Can you work these out from the model? Positions are in its coordinate system, mm. A direction names the side the tool comes from. Round coordinates to 2 decimals unless told otherwise and drop trailing zeros. Loops run counter-clockwise (first coordinate to the right, second up) from the corner with the lowest first, then second, coordinate; pieces in that order, holes last. Notation, with made-up numbers: (11.25, -1.5) -> (40.25, -1.5) arc R22 cw to (40.25, 35.5) -> close; hole circle Ø3 at (-37, 57). An arc over 180 degrees is marked (long way). Write each question's results on one line, items separated by ' | '.
from build123d import *

# Parameters (mm, degrees)
F0_R     = 17.5
F1_DEPTH = 4.9
F2_R     = 30
F3_DEPTH = 6.6
F4_SIZE  = 2
F5_R     = 7.5
F5_R_2   = 4.075
F6_DEPTH = 7.7
F7_DEPTH = 11.501


with BuildPart() as f1:
    # F0 (on Top) → F1 (new body)
    with BuildSketch(Plane.XY):
        Circle(F0_R)
    extrude(amount=F1_DEPTH)

    # F2 (on face) → F3 (join)
    with BuildSketch(Plane.XY.offset(4.9)):
        Circle(F2_R)
    extrude(amount=F3_DEPTH)

    # F4
    f4_edges = [f1.edges().sort_by_distance(p)[0] for p in [
        (-30, 0, 11.5),
    ]]
    chamfer(f4_edges, length=F4_SIZE)

    # F5 (on face) → F6 (cut)
    with BuildSketch(Plane.XY.offset(11.5)):
        with Locations((-8.8, 0)):
            Circle(F5_R)
        with Locations((-8.8, 0)):
            Circle(F5_R_2, mode=Mode.SUBTRACT)
        with Locations((8.8, 0)):
            Circle(F5_R)
        with Locations((8.8, 0)):
            Circle(F5_R_2, mode=Mode.SUBTRACT)
    extrude(amount=-F6_DEPTH, mode=Mode.SUBTRACT)

    # F7 (cut, through all): faces of the model
    f7_faces = [f1.faces().sort_by_distance(p)[0] for p in [
        (-8.8, 0, 11.5),
        (8.8, 0, 11.5),
    ]]
    extrude(f7_faces, amount=-F7_DEPTH, mode=Mode.SUBTRACT)


solid = f1.part
1. On a 3-axis mill with a long thin cutter (end or side, diameter ignored), from which of +Z, -Z, +X, -X, +Y, -Y can I reach the whole of each face in a straight line? I mean faces 1 (the face through (-29.97, 1.32, 7.17)), 2 (the face through (15.73, -2.87, 7.7)), 3 (the face through (13, -13, 4.9)). Say none if no direction works.
Final values:
face 1: +Z, -Z | face 2: +Z | face 3: -Z
2. If we section it at A-A (x = 0): List the corners of the cut face in (y, z) for me.
Final values:
outline: (-30, 4.9) -> (-17.5, 4.9) -> (-17.5, 0) -> (17.5, 0) -> (17.5, 4.9) -> (30, 4.9) -> (30, 9.5) -> (28, 11.5) -> (-28, 11.5) -> (-30, 9.5) -> close
3. If we section it at C-C (z = 8.25): List the corners of the cut face in (x, y) for me, then the cut area to 3 significant figures.
Final values:
outline: circle Ø60 at (0, 0); hole circle Ø15 at (-8.8, 0); hole circle Ø15 at (8.8, 0) | area: 2,470 mm2
4. If we section it at B-B (y = 0): List the corners of the cut face in (x, z) for me (3 decimals), then the cut area to 3 significant figures.
Final values:
outline: (-30, 4.9) -> (-17.5, 4.9) -> (-17.5, 0) -> (-12.875, 0) -> (-12.875, 3.8) -> (-16.3, 3.8) -> (-16.3, 11.5) -> (-28, 11.5) -> (-30, 9.5) -> close; (-4.725, 0) -> (4.725, 0) -> (4.725, 3.8) -> (1.3, 3.8) -> (1.3, 11.5) -> (-1.3, 11.5) -> (-1.3, 3.8) -> (-4.725, 3.8) -> close; (12.875, 0) -> (17.5, 0) -> (17.5, 4.9) -> (30, 4.9) -> (30, 9.5) -> (28, 11.5) -> (16.3, 11.5) -> (16.3, 3.8) -> (12.875, 3.8) -> close | area: 271 mm2
5. We'd pull the mould along X, two halves only. Please class faces 4 (the face through (-13.887, -10.648, 2.416)), 5 (the face through (12, -3, 3.8)), 6 (the face through (0, 0, 11.5)): pulls with the +X half, pulls with the -X half, needs draft (parallel to the pull), parting line crosses it, or undercut.
Final values:
face 4: parting line crosses it | face 5: undercut | face 6: needs draft
6. Will these pins go through, and if not, where does the flat tip stop? pin 1 (3 mm diameter, centred on x = 2, z = 7, fed in from -Y); pin 2 (3 mm diameter, centred on x = 6.5, z = 3, fed in from -Y); pin 3 (13 mm diameter, centred on x = -8.8, y = 0, fed in from +Z).
Final values:
pin 1: y = -30 | pin 2: y = -16.77 | pin 3: z = 3.8
7. Please list where these lines run through material, in increasing order: line 1 (X direction, y = -2.5, z = 6.25); line 2 (Y direction, x = 8.8, z = 10.25); line 3 (Z direction, x = -17.5, y = -4.5). Write a range as from..to.
Final values:
line 1: -29.9..-15.87, -1.73..1.73, 15.87..29.9 | line 2: -27.89..-7.5, 7.5..27.89 | line 3: 4.9..11.5
